from build123d import *

# Parameters (mm, degrees)
EXTRUDE_1_DEPTH     = 12
EXTRUDE_2_DEPTH     = 6
CUT_EXTRUDE_1_DEPTH = 5
SKETCH_6_R          = 0.6
EXTRUDE_5_DEPTH     = 10
SKETCH_3_R          = 2.5
CUT_EXTRUDE_2_DEPTH = 1


with BuildPart() as part:
    # 草图1 → 凸台-拉伸1 (new body)
    with BuildSketch(Plane.XY):
        Polygon((-11.5, 11.5), (11.5, 11.5), (11.5, 10.5), (16, 10.5), (16, 8.5), (11.5, 8.5), (11.5, -11.5), (-11.5, -11.5), (-11.5, 8.5), (-16, 8.5), (-16, 10.5), (-11.5, 10.5), align=None)
    extrude(amount=EXTRUDE_1_DEPTH)

    # 草图2 → 凸台-拉伸2 (add)
    with BuildSketch(Plane(origin=(0, 11.5, 0), x_dir=(1, 0, 0), z_dir=(0, 1, 0))):
        with BuildLine():
            ThreePointArc((0.020833333, -8.445144707), (11.5, -6), (0.020833333, -3.554855293))
            ThreePointArc((0.020833333, -3.554855293), (-3, -6), (0.020833333, -8.445144707))
        make_face()
    extrude(amount=EXTRUDE_2_DEPTH)

    # 草图4 → 切除-拉伸1 (cut)
    with BuildSketch(Plane(origin=(0, 10.5, 0), x_dir=(1, 0, 0), z_dir=(0, 1, 0))):
        with BuildLine():
            Line((16, -5.433355599), (14.823962452, -5.433355599))
            ThreePointArc((14.823962452, -5.433355599), (13.036198089, -5.933355599), (14.823962452, -6.433355599))
            Line((14.823962452, -6.433355599), (16, -6.433355599))
            Line((16, -6.433355599), (16, -5.433355599))
        make_face()
        with BuildLine():
            Line((-16, -5.433355599), (-14.823962452, -5.433355599))
            ThreePointArc((-14.823962452, -5.433355599), (-13.036198089, -5.933355599), (-14.823962452, -6.433355599))
            Line((-14.823962452, -6.433355599), (-16, -6.433355599))
            Line((-16, -6.433355599), (-16, -5.433355599))
        make_face()
    extrude(amount=-CUT_EXTRUDE_1_DEPTH, mode=Mode.SUBTRACT)

    # 草图6 → 凸台-拉伸5 (add)
    with BuildSketch(Plane(origin=(11.5, 0, 0), x_dir=(0, 0, -1), z_dir=(1, 0, 0))):
        with Locations((-6, -8.9)):
            Circle(SKETCH_6_R)
        with Locations((-7.5, -8.9)):
            Circle(SKETCH_6_R)
        with Locations((-4.5, -8.9)):
            Circle(SKETCH_6_R)
    extrude(amount=EXTRUDE_5_DEPTH)

    # 草图3 → 切除-拉伸2 (cut)
    with BuildSketch(Plane(origin=(0, 17.5, 0), x_dir=(1, 0, 0), z_dir=(0, 1, 0))):
        with Locations((5.5, -6)):
            Circle(SKETCH_3_R)
    extrude(amount=-CUT_EXTRUDE_2_DEPTH, mode=Mode.SUBTRACT)


solid = part.part
For this review, take the finished solid that the model builds, in its own axes (mm). A direction names the side the tool comes from. Coordinates: 2 decimals unless noted, no trailing zeros. Loops run counter-clockwise (first coordinate to the right, second up) from the corner with the lowest first, then second, coordinate; pieces in that order, holes last. Notation, with made-up numbers: (6.25, 62.5) - (31.25, 62.5) arc R18 ccw to (31.25, 79.5) - close; hole circle Ø9 at (72.5, 88.25). An arc over 180 degrees is marked (long way). Return JSON: item names as keys, results as strings.
Item 1: Take a section at A-A (x = 14). Give the boundary of the cut face in (y, z), then the cut area to 3 significant figures.
Determined:
{"outline": "circle Ø1.2 at (-8.9, 4.5); circle Ø1.2 at (-8.9, 6); circle Ø1.2 at (-8.9, 7.5); (8.5, 0) - (10.5, 0) - (10.5, 4.97) - (8.5, 4.97) - close; (8.5, 6.9) - (10.5, 6.9) - (10.5, 12) - (8.5, 12) - close", "area": "23.5 mm2"}
Item 2: Mouldability with a two-part tool opening along X and no side actions: class faces 1 (the flat face through (-16, 9, 3)), 2 (the flat face through (11.5, 11, 6)), 3 (the cylindrical face through (-13.037, 9.514, 5.898)), 4 (the flat face through (0, 0, 0)) as pulls with the +X half, pulls with the -X half, needs draft (parallel to the pull), parting line crosses it, or undercut.
Determined:
{"face 1": "pulls with the -X half", "face 2": "pulls with the +X half", "face 3": "undercut", "face 4": "needs draft"}
Item 3: Take a section at C-C (x = -0.5). Give the boundary of the cut face in (y, z).
Determined:
{"outline": "(-11.5, 0) - (11.5, 0) - (11.5, 3.5) - (17.5, 3.5) - (17.5, 8.5) - (11.5, 8.5) - (11.5, 12) - (-11.5, 12) - close"}
Item 4: Insertion check: pin 1 (5 mm diameter, centred on y = -5, z = 5.5, fed in from +X); pin 2 (2.5 mm diameter, centred on x = -14, z = 5.93, fed in from +Y); pin 3 (5 mm diameter, centred on x = -14.5, z = 8, fed in from -Y). Each pin has a flat end and moves straight along its axis. Give the tip position at first contact, or say it passes through.
Determined:
{"pin 1": "stops at x = 11.5", "pin 2": "stops at y = 10.5", "pin 3": "stops at y = 8.5"}
Item 5: Take a section at B-B (y = -8.9). Give the boundary of the cut face in (x, z).
Determined:
{"outline": "(-11.5, 0) - (11.5, 0) - (11.5, 3.9) - (21.5, 3.9) - (21.5, 5.1) - (11.5, 5.1) - (11.5, 5.4) - (21.5, 5.4) - (21.5, 6.6) - (11.5, 6.6) - (11.5, 6.9) - (21.5, 6.9) - (21.5, 8.1) - (11.5, 8.1) - (11.5, 12) - (-11.5, 12) - close"}
Item 6: For faces 5 (the flat face through (-15, 10, 5.433)), 6 (the flat face through (12.8, 8.5, 5.9)), 7 (the flat face through (10, 11.5, 1)), list the 3-axis set-ups (+Z, -Z, +X, -X, +Y, -Y) from which the entire face can be reached by the end or side of a thin tool; tool diameter is ignored.
Determined:
{"face 5": "-X, +Y, -Y", "face 6": "+Z, -Z, +X", "face 7": "-Z, +X, +Y"}
Item 7: For line 1 (Z direction, x = 14, y = 9.7); line 2 (Z direction, x = 5.5, y = 17.25); line 3 (X direction, y = 7.75, z = 5.5), list the stretches that pass through material, from the lowest coordinate up.
Determined:
{"line 1": "z = 0 to 4.97, 6.9 to 12", "line 2": "z = 0 to 3.5, 8.5 to 12", "line 3": "x = -11.5 to 11.5"}
Item 8: Take a section at D-D (z = 9). Give the boundary of the cut face in (x, y), then the cut area to 3 significant figures.
Determined:
{"outline": "(-16, 8.5) - (-11.5, 8.5) - (-11.5, -11.5) - (11.5, -11.5) - (11.5, 8.5) - (16, 8.5) - (16, 10.5) - (11.5, 10.5) - (11.5, 11.5) - (10.7, 11.5) - (10.7, 17.5) - (0.3, 17.5) - (0.3, 11.5) - (-11.5, 11.5) - (-11.5, 10.5) - (-16, 10.5) - close", "area": "609 mm2"}
